Could you check a few things on this drawing? It's one solid part, dimensions in mm from its lowest x, y, z. Give positions to 0.01 mm unless a question says otherwise; leave off trailing zeros. Order: outer loops, then holes, each group sorted by start corner. A loop starts at its lowest first (then second) coordinate and runs counter-clockwise, first axis right, second up. Notation, with made-up numbers: (25, 30) - (35, 30) arc R27 ccw to (35, 51) - close; hole circle Ø3 at (39, -30.5). An arc over 180 degrees is marked (long way). Put each result on its own line as item: value.
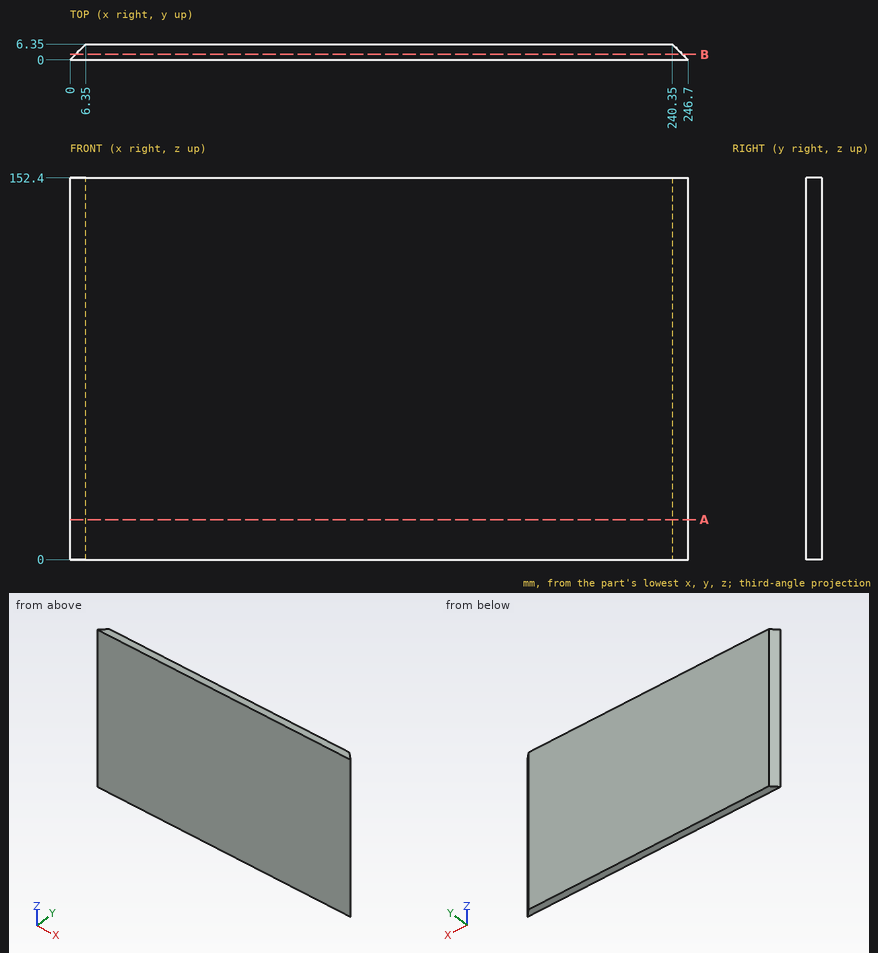
1) If I drill on line 1 (X direction, y = 3.75, z = 102); line 2 (X direction, y = 2.5, z = 123), over which ranges is the centre line in solid material (lowest first)? Write a range as [from, to].
Filled in:
line 1: x = [3.75, 242.95]
line 2: x = [2.5, 244.2]
2) I'm going to push flat-ended pins straight in: pin 1 (2 mm diameter, centred on y = 1.5, z = 70.5, fed in from +X); pin 2 (2 mm diameter, centred on y = 2, z = 81.5, fed in from +X). Where does each tip first touch, or does it pass through?
Filled in:
pin 1: stops at x = 246.2
pin 2: stops at x = 245.7
3) Suppose I cut it at A-A, the plane z = 16. List the corners of the cut face in (x, y) for me.
Filled in:
outline: (0, 0) - (246.7, 0) - (240.35, 6.35) - (6.35, 6.35) - close
4) Suppose I cut it at B-B, the plane y = 2.25. List the corners of the cut face in (x, z) for me, and give its area (3 significant figures).
Filled in:
outline: (2.25, 0) - (244.45, 0) - (244.45, 152.4) - (2.25, 152.4) - close
area: 36,900 mm^2
